Design review of the part built by this model. Coordinates are the model's own, in mm. A direction names the side the tool comes from. Round coordinates to 2 decimals unless told otherwise and drop trailing zeros. Loops run counter-clockwise (first coordinate to the right, second up) from the corner with the lowest first, then second, coordinate; pieces in that order, holes last. Notation, with made-up numbers: M 45.5,52 L 61.5,52 A17 cw 61.5,68 Z; hole C -11.75,87 d7. An arc over 180 degrees is marked long. One line per item, written item: value. Start each with the question number.
Item 1: Clearance check with flat-ended pins moving along their axes: pin 1 (3 mm diameter, centred on x = -52.38, y = -3.72, fed in from -Z); pin 2 (1 mm diameter, centred on x = -53, z = 2.5, fed in from +Y); pin 3 (1.8 mm diameter, centred on x = -52, y = -2.5, fed in from +Z). State where each tip first meets the part, or that it passes through.
Item 2: We need section D-D (x = -49.9). Write out the cut boundary in (y, z), then the cut area to 3 significant figures.
Item 3: We need section A-A (y = 7.5). Write out the cut boundary in (x, z).
Item 4: We need section C-C (z = 2.1). Write out the cut boundary in (x, y).
Item 5: Mouldability with a two-part tool opening along Y and no side actions: class faces 1 (the cylindrical face through (-51.421, 8.075, 0.386)), 2 (the cylindrical face through (-49.676, 4.74, 3.022)), 3 (the cylindrical face through (-51.421, -3.425, 0.386)), 4 (the flat face through (-55.375, 2, 1)) as released by +Y, released by -Y, zero draft, split by the parting line, or undercut.
Item 6: We need section B-B (x = -52.9). Write out the cut boundary in (y, z).
Item 7: For faces 5 (the cylindrical face through (-55.09, 4.724, 3.022)), 6 (the cylindrical face through (-55.09, -0.674, 3.022)), 7 (the cylindrical face through (-49.676, -0.69, 3.022)), list the 3-axis set-ups (+Z, -Z, +X, -X, +Y, -Y) from which the entire face can be reached by the end or side of a thin tool; tool diameter is ignored.
Item 8: For line 1 along X through (y, z) = (-3.75, 0.5); line 2 along Z through (x, y) = (-54.1, 7.5); line 3 along Y through (x, z) = (-52.25, 3.15), list the stretches that pass through material, from the lowest coordinate up.
from build123d import *

# Parameters (mm, degrees)
SKETCH043_W  = 6
SKETCH043_H  = 17.5
SKETCH043_R  = 1
PAD017_DEPTH = 2
SKETCH044_W  = 6
SKETCH044_H  = 6
PAD018_DEPTH = 3.2
FILLET_R     = 2.9
FILLET001_R  = 1


with BuildPart() as part:
    # Sketch043 (on DatumPlane) → Pad017 (new body)
    with BuildSketch(Plane.XY.offset(-0.600022)):
        with Locations((-52.375043, 2.025062)):
            Rectangle(SKETCH043_W, SKETCH043_H)
        with Locations((-52.375043, 7.775062)):
            Circle(SKETCH043_R, mode=Mode.SUBTRACT)
        with Locations((-52.375043, -3.724938)):
            Circle(SKETCH043_R, mode=Mode.SUBTRACT)
    extrude(amount=PAD017_DEPTH)

    # Sketch044 (on Face8 of Pad017) → Pad018 (join)
    with BuildSketch(Plane.XY.offset(1.399978)):
        with Locations((-52.375043, 2.025062)):
            Rectangle(SKETCH044_W, SKETCH044_H)
    extrude(amount=PAD018_DEPTH)

    # Fillet
    fillet_edges = [part.edges().sort_by_distance(p)[0] for p in [
        (-49.375043, 10.775062, 0.399978),
        (-55.375043, 10.775062, 0.399978),
        (-49.375043, -6.724938, 0.399978),
        (-55.375043, -6.724938, 0.399978),
    ]]
    fillet(fillet_edges, radius=FILLET_R)

    # Fillet001
    fillet001_edges = [part.edges().sort_by_distance(p)[0] for p in [
        (-49.375043, -0.974938, 2.999978),
        (-55.375043, -0.974938, 2.999978),
        (-49.375043, 5.025062, 2.999978),
        (-55.375043, 5.025062, 2.999978),
    ]]
    fillet(fillet001_edges, radius=FILLET001_R)


solid = part.part
A:
1. pin 1: z = -0.6
1. pin 2: y = 5.03
1. pin 3: z = 1.4
2. outline: M -5.49,-0.6 L 9.54,-0.6 L 9.54,1.4 L 4.91,1.4 L 4.91,4.6 L -0.85,4.6 L -0.85,1.4 L -5.49,1.4 Z
2. area: 48.5 mm2
3. outline: M -55.38,-0.6 L -53.34,-0.6 L -53.34,1.4 L -55.38,1.4 Z; M -51.41,-0.6 L -49.38,-0.6 L -49.38,1.4 L -51.41,1.4 Z
4. outline: M -55.38,0.03 A1 ccw -54.38,-0.97 L -50.38,-0.97 A1 ccw -49.38,0.03 L -49.38,4.03 A1 ccw -50.38,5.03 L -54.38,5.03 A1 ccw -55.38,4.03 Z
5. face 1: undercut
5. face 2: released by +Y
5. face 3: undercut
5. face 4: zero draft
6. outline: M -6.69,-0.6 L -4.58,-0.6 L -4.58,1.4 L -6.69,1.4 Z; M -2.87,-0.6 L 6.92,-0.6 L 6.92,1.4 L 5.03,1.4 L 5.03,4.6 L -0.97,4.6 L -0.97,1.4 L -2.87,1.4 Z; M 8.63,-0.6 L 10.74,-0.6 L 10.74,1.4 L 8.63,1.4 Z
7. face 5: +Z, -X, +Y
7. face 6: +Z, -X, -Y
7. face 7: +Z, +X, -Y
8. line 1: -55.38 to -53.37, -51.38 to -49.38
8. line 2: -0.6 to 1.4
8. line 3: -0.97 to 5.03
